Verification items for the finished model (mm, model axes). Give positions to 0.01 mm unless a question says otherwise; leave off trailing zeros. Loops run counter-clockwise (first coordinate to the right, second up) from the corner with the lowest first, then second, coordinate; pieces in that order, holes last. Notation, with made-up numbers: M -1.75,80 L 21.25,80 A26 ccw 21.25,95 Z; hole C 27,5.5 d3. An arc over 180 degrees is marked long. Use CSV: the item, a comma, the result in double quotes.
from build123d import *

# Parameters (mm, degrees)
SKETCH1_R      = 4
EXTRUDE1_DEPTH = 20
CHAMFER2_SIZE  = 3
CHAMFER2_SIZE2 = 1.091910703
CHAMFER3_SIZE  = 3
CHAMFER3_SIZE2 = 1.091910703


with BuildPart() as part:
    # Sketch1 → Extrude1 (new body)
    with BuildSketch(Plane.XY):
        Circle(SKETCH1_R)
    extrude(amount=EXTRUDE1_DEPTH)

    # Chamfer2
    chamfer2_edges = [part.edges().sort_by_distance(p)[0] for p in [
        (-4, 0, 20),
    ]]
    chamfer2_side = [part.faces().sort_by_distance(p)[0] for p in [
        (-4, 0, 10),
    ]]
    chamfer(chamfer2_edges, length=CHAMFER2_SIZE, length2=CHAMFER2_SIZE2, reference=chamfer2_side[0])

    # Chamfer3
    chamfer3_edges = [part.edges().sort_by_distance(p)[0] for p in [
        (-4, 0, 0),
    ]]
    chamfer3_side = [part.faces().sort_by_distance(p)[0] for p in [
        (-4, 0, 8.5),
    ]]
    chamfer(chamfer3_edges, length=CHAMFER3_SIZE, length2=CHAMFER3_SIZE2, reference=chamfer3_side[0])


solid = part.part
(1) Section check C-C on z = 16.5. Record the cut outline in (x, y), plus the area to 3 significant figures.
Calculated:
outline,"C 0,0 d8"
area,"50.3 mm²"
(2) Scan lines: L1, parallel to Y at x = 2.75, z = 10.25; L2, parallel to Z at x = -2.75, y = 2; L3, parallel to X at y = 3.5, z = 16. Record each from-to range of solid material in increasing order. Write a range as from..to.
Calculated:
L1,"y = -2.9..2.9"
L2,"z = 1.35..18.65"
L3,"x = -1.94..1.94"
(3) Section check A-A on x = 0. Record the cut outline in (y, z), plus the area to 3 significant figures.
Calculated:
outline,"M -4,3 L -2.91,0 L 2.91,0 L 4,3 L 4,17 L 2.91,20 L -2.91,20 L -4,17 Z"
area,"153 mm²"
(4) Depth check by flat-ended pin: pin 1 Ø1.5 at (x, z) = (1.5, 16.5) entering from +Y. Enter the tip coordinate at first touch or a pass-through.
Calculated:
pin 1,"stops at y = 3.93"
